Check sheet for the modelled part. Datum: model origin and axes. Units: mm. Face numbers are marked on the shaded views. A direction names the side the tool comes from. Give positions to 0.01 mm unless a question says otherwise; leave off trailing zeros. Loops run counter-clockwise (first coordinate to the right, second up) from the corner with the lowest first, then second, coordinate; pieces in that order, holes last. Notation, with made-up numbers: (-36, -17) -> (11, -17) arc R28 cw to (11, 10) -> close; hole circle Ø3 at (-36, 9). An arc over 180 degrees is marked (long way). Write each question's results on one line, items separated by ' | '. Start each with the question number.
Item 1: Scan lines: line 1 along Z through (x, y) = (-1.15, -0.5); line 2 along Z through (x, y) = (-0.65, 2.05); line 3 along Y through (x, z) = (-0.75, -0.75). Record each from-to range of solid material in increasing order.
Item 2: Cross-section at A-A on z = 0.75. Enter the section's corners in (x, y), then the cut area to 3 significant figures.
Item 3: Access from +Z, -Z, +X, -X, +Y, -Y to the whole of each face (thin tool, end or side, straight path). Record for the marked faces 4, 5 and 6.
Item 4: Mould release check, pull along X, two halves, no side actions. Record for the marked faces 1, 2 and 3: pulls with the +X half, pulls with the -X half, needs draft (parallel to the pull), parting line crosses it, or undercut.
Item 5: Cross-section at B-B on z = -2. Enter the section's corners in (x, y) (1 decimal), then the cut area to 3 significant figures.
Item 6: Gauge pin test, flat ends, axial feed: pin 1 Ø0.6 at (x, y) = (-1, 0.5) entering from -Z; pin 2 Ø1.5 at (x, y) = (-2, -2) entering from -Z. Record the tip position at first contact, or that the pin passes through.
from build123d import *

# Parameters (mm, degrees)
FILLET1_R          = 0.1
FILLET2_R          = 0.25
HOLE1_D            = 2.05
HOLE1_DEPTH        = 1
HOLE1_TIP          = 0.37306949
CUT_EXTRUDE1_DEPTH = 1


with BuildPart() as part:
    # Sketch1 → Base-Revolve (revolve)
    with BuildSketch(Plane(origin=(0, 0, 0), x_dir=(0, 0, -1), z_dir=(1, 0, 0))):
        with BuildLine():
            Line((-5, 0), (-5, 1.5))
            Line((-5, 1.5), (0, 1.5))
            Line((0, 1.5), (0, 2.8))
            Line((0, 2.8), (1, 2.8))
            ThreePointArc((1, 2.8), (1.799098682, 2.280109646), (2.4, 1.54))
            Line((2.4, 1.54), (2.4, 0))
            Line((2.4, 0), (-5, 0))
        make_face()
    revolve(axis=Axis((0, 0, -2.4), (0, 0, 1)))

    # Fillet1
    fillet1_edges = [part.edges().sort_by_distance(p)[0] for p in [
        (0, -1.5, 0),
    ]]
    fillet(fillet1_edges, radius=FILLET1_R)

    # Fillet2
    fillet2_edges = [part.edges().sort_by_distance(p)[0] for p in [
        (0, -2.8, -1),
        (0, -2.8, 0),
    ]]
    fillet(fillet2_edges, radius=FILLET2_R)

    # Hole1
    with Locations(Plane(origin=(0, 0, -2.4), x_dir=(-1, 0, 0), z_dir=(0, 0, -1))):
        with Locations((0, 0)):
            Hole(HOLE1_D / 2, depth=HOLE1_DEPTH)
            with Locations((0, 0, -(HOLE1_DEPTH + HOLE1_TIP / 2))):  # 140° drill point
                Cone(0, HOLE1_D / 2, HOLE1_TIP, mode=Mode.SUBTRACT)

    # Sketch4 → Cut-Extrude1 (cut)
    with BuildSketch(Plane(origin=(0, 0, -2.4), x_dir=(-1, 0, 0), z_dir=(0, 0, -1))):
        with BuildLine():
            ThreePointArc((1.088832331, -0.880025088), (1.212435565, -0.7), (1.306540248, -0.502943915))
            ThreePointArc((1.306540248, -0.502943915), (1.025, 0), (1.306540248, 0.502943915))
            ThreePointArc((1.306540248, 0.502943915), (1.212435565, 0.7), (1.088832331, 0.880025088))
            ThreePointArc((1.088832331, 0.880025088), (0.5125, 0.887676039), (0.217707917, 1.382969003))
            ThreePointArc((0.217707917, 1.382969003), (0, 1.4), (-0.217707917, 1.382969003))
            ThreePointArc((-0.217707917, 1.382969003), (-0.5125, 0.887676039), (-1.088832331, 0.880025088))
            ThreePointArc((-1.088832331, 0.880025088), (-1.212435565, 0.7), (-1.306540248, 0.502943915))
            ThreePointArc((-1.306540248, 0.502943915), (-1.025, 0), (-1.306540248, -0.502943915))
            ThreePointArc((-1.306540248, -0.502943915), (-1.212435565, -0.7), (-1.088832331, -0.880025088))
            ThreePointArc((-1.088832331, -0.880025088), (-0.5125, -0.887676039), (-0.217707917, -1.382969003))
            ThreePointArc((-0.217707917, -1.382969003), (0, -1.4), (0.217707917, -1.382969003))
            ThreePointArc((0.217707917, -1.382969003), (0.5125, -0.887676039), (1.088832331, -0.880025088))
        make_face()
    extrude(amount=-CUT_EXTRUDE1_DEPTH, mode=Mode.SUBTRACT)


solid = part.part
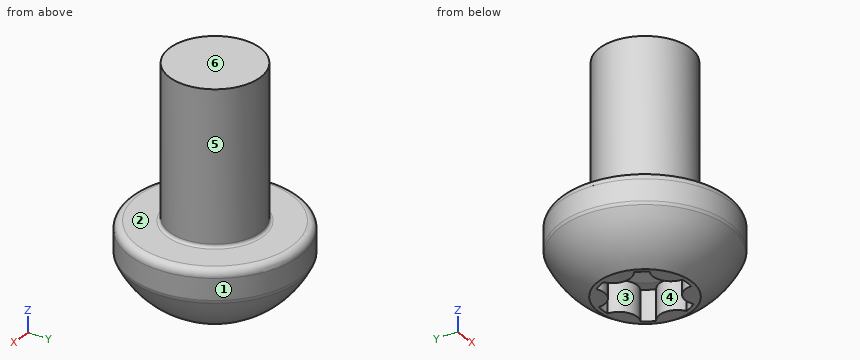
Answer sheet:
1) line 1: z = -1.4 to 5 | line 2: z = -1.93 to 0 | line 3: y = -2.7 to 2.7
2) outline: circle Ø3 at (0, 0) | area: 7.07 mm²
3) face 4: -Z | face 5: +Z | face 6: +Z, +X, -X, +Y, -Y
4) face 1: parting line crosses it | face 2: needs draft | face 3: undercut
5) outline: circle Ø4.2 at (0, 0); hole (-1.3, -0.5) arc R1.4 ccw to (-1.1, -0.9) arc R0.6 cw to (-0.2, -1.4) arc R1.4 ccw to (0.2, -1.4) arc R0.6 cw to (1.1, -0.9) arc R1.4 ccw to (1.3, -0.5) arc R0.6 cw to (1.3, 0.5) arc R1.4 ccw to (1.1, 0.9) arc R0.6 cw to (0.2, 1.4) arc R1.4 ccw to (-0.2, 1.4) arc R0.6 cw to (-1.1, 0.9) arc R1.4 ccw to (-1.3, 0.5) arc R0.6 cw to start | area: 9.04 mm²
6) pin 1: stops at z = -2.4 | pin 2: stops at z = -2
